The drawing under review shows one solid part. Ordinate dimensions are in mm from its lowest x, y, z. A direction names the side the tool comes from. Round coordinates to 2 decimals unless told otherwise and drop trailing zeros. Order: outer loops, then holes, each group sorted by start corner. A loop starts at its lowest first (then second) coordinate and runs counter-clockwise, first axis right, second up. Notation, with made-up numbers: M 2.5,23.5 L 59.5,23.5 A12 cw 59.5,28.5 Z; hole C 48,57.5 d7. An arc over 180 degrees is marked long. Write item = value, one per line. Start each with the question number.
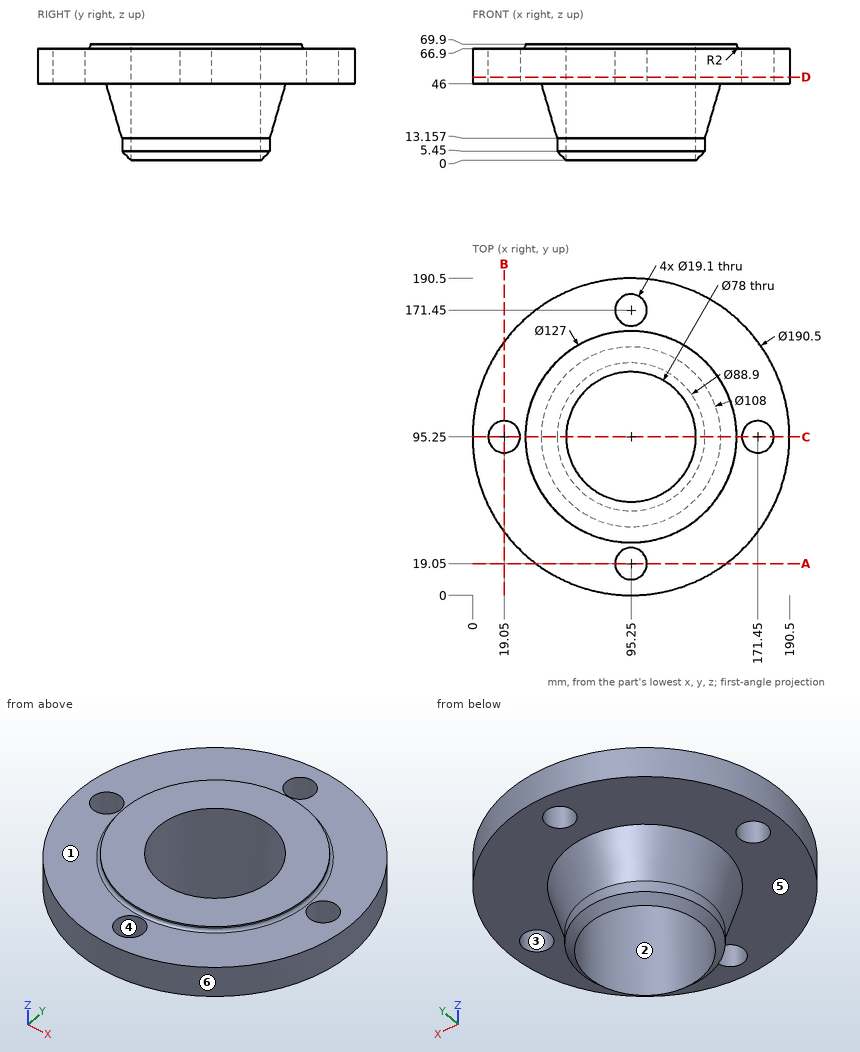
(1) Consider section C-C, the plane y = 95.25. Write out the cut boundary in (x, z).
(2) Draft analysis for pull direction Y (two halves, no side actions). For the marked faces 3, 4, 5 and 6, state which applies: pulls with the +Y half, pulls with the -Y half, needs draft (parallel to the pull), parting line crosses it, or undercut.
(3) Consider section A-A, the plane y = 19.05. Write out the cut boundary in (x, z).
(4) Insertion check: pin 1 (25 mm diameter, centred on x = 19.05, y = 95.25, fed in from -Z); pin 2 (5 mm diameter, centred on x = 78, z = 30, fed in from -Y); pin 3 (1 mm diameter, centred on y = 77, z = 57, fed in from +X); pin 4 (6 mm diameter, centred on x = 79.5, y = 133.5, fed in from -Z). Each pin has a flat end and moves straight along its axis. Give the tip position at first contact, or say it passes through.
(5) For the marked faces 1 and 2, list the 3-axis set-ups (+Z, -Z, +X, -X, +Y, -Y) from which the entire face can be reached by the end or side of a thin tool; tool diameter is ignored.
(6) For line 1 along Y through (x, z) = (95.25, 57.5); line 2 along Z through (x, y) = (159, 156.5); line 3 along Z through (x, y) = (60, 145), list the stretches that pass through material, from the lowest coordinate up. Write a range as [from, to].
(7) Consider section D-D, the plane z = 50. Write out the cut boundary in (x, y), then the cut area to 3 significant figures.
Completed:
q1.outline = M 0,46 L 9.5,46 L 9.5,66.9 L 0,66.9 Z; M 28.6,46 L 41.25,46 L 50.8,13.16 L 50.8,5.45 L 56.25,0 L 56.25,69.9 L 31.75,69.9 L 31.75,68.9 A2 cw 29.75,66.9 L 28.6,66.9 Z; M 134.25,0 L 139.7,5.45 L 139.7,13.16 L 149.25,46 L 161.9,46 L 161.9,66.9 L 160.75,66.9 A2 cw 158.75,68.9 L 158.75,69.9 L 134.25,69.9 Z; M 181,46 L 190.5,46 L 190.5,66.9 L 181,66.9 Z
q2.face_3 = undercut
q2.face_4 = undercut
q2.face_5 = needs draft
q2.face_6 = parting line crosses it
q3.outline = M 38.1,46 L 85.7,46 L 85.7,66.9 L 38.1,66.9 Z; M 104.8,46 L 152.4,46 L 152.4,66.9 L 104.8,66.9 Z
q4.pin_1 = 46
q4.pin_2 = 47.85
q4.pin_3 = 188.83
q4.pin_4 = 0
q5.face_1 = +Z
q5.face_2 = +Z, -Z
q6.line_1 = [0, 9.5], [28.6, 56.25], [134.25, 161.9], [181, 190.5]
q6.line_2 = [46, 66.9]
q6.line_3 = [46, 69.9]
q7.outline = C 95.25,95.25 d190.5; hole C 19.05,95.25 d19.1; hole C 95.25,95.25 d78; hole C 95.25,19.05 d19.1; hole C 95.25,171.45 d19.1; hole C 171.45,95.25 d19.1
q7.area = 22,600 mm2
